from build123d import *

# Parameters (mm, degrees)
SKETCH1_R           = 1.6
BOSS_EXTRUDE1_DEPTH = 2
FILLET1_R           = 4


with BuildPart() as part:
    # Sketch1 → Boss-Extrude1 (new body)
    with BuildSketch(Plane.XY):
        with BuildLine():
            Line((-32.992640687, -24.6), (-26.492640687, -31.1))
            Line((-26.492640687, -31.1), (-5.656854249, -31.1))
            Line((-5.656854249, -31.1), (1.671572875, -38.428427125))
            ThreePointArc((1.671572875, -38.428427125), (7.328427125, -38.428427125), (7.328427125, -32.771572875))
            Line((7.328427125, -32.771572875), (-8.843145751, -16.6))
            Line((-8.843145751, -16.6), (-55, -16.6))
            ThreePointArc((-55, -16.6), (-59, -20.6), (-55, -24.6))
            Line((-55, -24.6), (-32.992640687, -24.6))
        make_face()
        with Locations((-25.25, -28.1)):
            Circle(SKETCH1_R, mode=Mode.SUBTRACT)
        with Locations((4.5, -35.6)):
            Circle(SKETCH1_R, mode=Mode.SUBTRACT)
        with Locations((-55, -20.6)):
            Circle(SKETCH1_R, mode=Mode.SUBTRACT)
    extrude(amount=BOSS_EXTRUDE1_DEPTH)

    # Fillet1
    fillet1_edges = [part.edges().sort_by_distance(p)[0] for p in [
        (-8.843145751, -16.6, 1),
        (-5.656854249, -31.1, 1),
        (-26.492640687, -31.1, 1),
        (-32.992640687, -24.6, 1),
    ]]
    fillet(fillet1_edges, radius=FILLET1_R)


solid = part.part
Can you work these out from the model? Positions are in its coordinate system, mm. A direction names the side the tool comes from. Coordinates: 2 decimals unless noted, no trailing zeros. Loops run counter-clockwise (first coordinate to the right, second up) from the corner with the lowest first, then second, coordinate; pieces in that order, holes last. Notation, with made-up numbers: (57, 29.5) - (71, 29.5) arc R31 ccw to (71, 53.5) - close; hole circle Ø3 at (74, -14). An arc over 180 degrees is marked (long way). Put each result on its own line as item: value. Start each with the question number.
Item 1: Suppose I cut it at D-D (x = -12). Please give me the cut outline in (y, z).
Item 2: Which directions (+Z, -Z, +X, -X, +Y, -Y) give clear straight access to the entire face, cutting with the end or side of a thin tool? Please do faces 5 (the face through (-45, -24.6, 1)), 6 (the face through (-32, -16.6, 1)).
Item 3: If we mould it in two halves opening along X, with no side actions, what happens to faces 1 (the face through (-8.99, -16.896, 1.014)), 2 (the face through (-59, -20.5, 1)), 3 (the face through (-25.6, -29.66, 0.99)), 4 (the face through (5.24, -37.02, 0.99))? For each: +X half, -X half, draft (parallel to the pull), parting line (faces both ways), or undercut.
Item 4: If I drill on line 1 along Y through (x, z) = (-55, 1); line 2 along Y through (x, z) = (4.5, 1.65); line 3 along Y through (x, z) = (-19.5, 0.55), over which ranges is the centre line in solid material (lowest first)?
Item 5: Suppose I cut it at A-A (z = 1.2). Please give me the cut outline in (x, y), and give its area (3 significant figures).
Item 6: Suppose I cut it at C-C (y = -35.6). Please give me the cut outline in (x, z).
Item 7: For pin 1 (1 mm diameter, centred on x = -45, z = 1, fed in from -Y), with a flat end and sliding along its axis, tell me the tip position at first contact or that it passes through.
Item 8: Suppose I cut it at B-B (x = -54). Please give me the cut outline in (y, z), and give its area (3 significant figures).
Here are the results:
1. outline: (-31.1, 0) - (-16.6, 0) - (-16.6, 2) - (-31.1, 2) - close
2. face 5: +Z, -Z, -X, -Y
2. face 6: +Z, -Z, +X, -X, +Y
3. face 1: +X half
3. face 2: -X half
3. face 3: undercut
3. face 4: undercut
4. line 1: -24.6 to -22.2, -19 to -16.6
4. line 2: -39.6 to -37.2, -34 to -29.94
4. line 3: -31.1 to -16.6
5. outline: (-55, -24.6) - (-34.65, -24.6) arc R4 cw to (-31.82, -25.77) - (-27.66, -29.93) arc R4 ccw to (-24.84, -31.1) - (-7.31, -31.1) arc R4 cw to (-4.49, -32.27) - (1.67, -38.43) arc R4 ccw to (7.33, -32.77) - (-7.67, -17.77) arc R4 ccw to (-10.5, -16.6) - (-55, -16.6) arc R4 ccw to start; hole circle Ø3.2 at (-55, -20.6); hole circle Ø3.2 at (-25.25, -28.1); hole circle Ø3.2 at (4.5, -35.6)
5. area: 687 mm²
6. outline: (-1.16, 0) - (2.9, 0) - (2.9, 2) - (-1.16, 2) - close; (6.1, 0) - (8.5, 0) - (8.5, 2) - (6.1, 2) - close
7. pin 1: y = -24.6
8. outline: (-24.6, 0) - (-21.85, 0) - (-21.85, 2) - (-24.6, 2) - close; (-19.35, 0) - (-16.6, 0) - (-16.6, 2) - (-19.35, 2) - close
8. area: 11.0 mm²
